```python
from build123d import *

# Parameters (mm, degrees)
BOSS_EXTRUDE1_DEPTH = 12
SKETCH2_R           = 4.25
SKETCH2_R_2         = 1.6
CUT_EXTRUDE2_DEPTH  = 13


with BuildPart() as part:
    # Sketch1 → Boss-Extrude1 (new body)
    with BuildSketch(Plane.XY):
        Polygon((-14, 0), (14, 0), (9.8, 48), (-9.8, 48), align=None)
    extrude(amount=BOSS_EXTRUDE1_DEPTH)

    # Sketch2 → Cut-Extrude2 (cut)
    with BuildSketch(Plane.XY):
        with Locations((0, 28)):
            Circle(SKETCH2_R)
        with Locations((10, 6)):
            Circle(SKETCH2_R_2)
        with Locations((-10, 6)):
            Circle(SKETCH2_R_2)
    extrude(amount=CUT_EXTRUDE2_DEPTH, mode=Mode.SUBTRACT)


solid = part.part
```
Here's how the part is built. I have some questions about the finished solid (model axes, mm). Round coordinates to 2 decimals unless told otherwise and drop trailing zeros. Write each loop counter-clockwise with the first axis right and the second up, starting at its lowest first coordinate (ties: lowest second). Pieces come first, ordered by that corner, then holes.
Q1. If we mould it in two halves opening along Y, with no side actions, what happens to faces 1 (the flat face through (0, 0, 6)), 2 (the flat face through (0, 48, 6)), 3 (the cylindrical face through (2.285, 31.584, 5.916))? For each: +Y half, -Y half, draft (parallel to the pull), parting line (faces both ways), or undercut.
Q2. Please list where these lines run through material, in increasing order: probe 1 along X at (y, z) = (6, 3) (3 decimals); probe 2 along X at (y, z) = (28, 7.25); probe 3 along Y at (x, z) = (0, 8).
Q3. If we section it at D-D on y = 11: Write out the boundary of the cut face in (x, z).
Q4. If we section it at B-B on z = 2.75: Write out the boundary of the cut face in (x, y), plus the area to 3 significant figures.
Q5. If we section it at C-C on y = 27: Write out the boundary of the cut face in (x, z), plus the area to 3 significant figures.
Q6. Will these pins go through, and if not, where does the flat tip stop? P1, Ø3, axis at y = 23.5, z = 3, coming from the -X side (3 decimals); P2, Ø1.5, axis at y = 5, z = 7.5, coming from the +X side; P3, Ø3, axis at y = 31.5, z = 5, coming from the -X side (3 decimals).
Q7. If we section it at A-A on x = 0: Write out the boundary of the cut face in (y, z).
Answer below:
1. face 1: -Y half
1. face 2: +Y half
1. face 3: undercut
2. probe 1: x = -13.475 to -11.6, -8.4 to 8.4, 11.6 to 13.475
2. probe 2: x = -11.55 to -4.25, 4.25 to 11.55
2. probe 3: y = 0 to 23.75, 32.25 to 48
3. outline: (-13.04, 0) - (13.04, 0) - (13.04, 12) - (-13.04, 12) - close
4. outline: (-14, 0) - (14, 0) - (9.8, 48) - (-9.8, 48) - close; hole circle Ø3.2 at (-10, 6); hole circle Ø8.5 at (0, 28); hole circle Ø3.2 at (10, 6)
4. area: 1,070 mm2
5. outline: (-11.64, 0) - (-4.13, 0) - (-4.13, 12) - (-11.64, 12) - close; (4.13, 0) - (11.64, 0) - (11.64, 12) - (4.13, 12) - close
5. area: 180 mm2
6. P1: stops at x = -12.075
6. P2: stops at x = 13.63
6. P3: stops at x = -11.375
7. outline: (0, 0) - (23.75, 0) - (23.75, 12) - (0, 12) - close; (32.25, 0) - (48, 0) - (48, 12) - (32.25, 12) - close
